Autodesk Inventor part; units mm, degrees
ref_plane "YZ Plane" through (0, 0, 0) normal (1, 0, 0) x (0, 1, 0)
ref_plane "XZ Plane" through (0, 0, 0) normal (0, 1, 0) x (-1, 0, 0)
ref_plane "XY Plane" through (0, 0, 0) normal (0, 0, 1) x (1, 0, 0)
sketch "Sketch1" plane through (0, 0, 0) normal (0, 0, 1) x (0, 1, 0)
  circle A0 centre (103.8572, -128.4288) radius 17.5
  circle A1 centre (-46.1428, 47.5712) radius 30
  circle A2 centre (-36.5428, 154.0712) radius 17.5
  arc A3 (-12.2627, 179.2798) -> (-68.6436, 140.1233) centre (-36.5428, 154.0712) ccw
  arc A4 (-79.1765, 78.1289) -> (-52.7383, 3.0571) centre (-46.1428, 47.5712) ccw
  arc A5 (68.91, -130.351) -> (138.7018, -131.7234) centre (103.8572, -128.4288) ccw
  arc A6 (239.3875, 30.5679) -> (230.7678, 67.4797) centre (228.8572, 47.5712) ccw
  arc A7 (-79.1765, 78.1289) -> (-68.6436, 140.1233) centre (-121.4095, 117.1964) ccw
  arc A8 (68.91, -130.351) -> (-52.7383, 3.0571) centre (-73.6667, -138.1931) ccw
  arc A9 (239.3875, 30.5679) -> (138.7018, -131.7234) centre (352.4092, -151.9293) ccw
  arc A10 (-12.2627, 179.2798) -> (230.7678, 67.4797) centre (269.5808, 471.9005) ccw
  dimension "d0" = 106.5
  dimension "d1" = 176
  dimension "d2" = 150
  dimension "d3" = 9.6
  dimension "d4" = 275
  dimension "d5" = 60
  dimension "d6" = 35
  dimension "d7" = 35
  dimension "d8" = 35
  dimension "d9" = 35
  dimension "d10" = 45
  dimension "d11" = 20
extrude "Extrusion1" add sketch "Sketch1" along normal blind 10
properties part number "3136 1133 85" material "Steel, Mild"
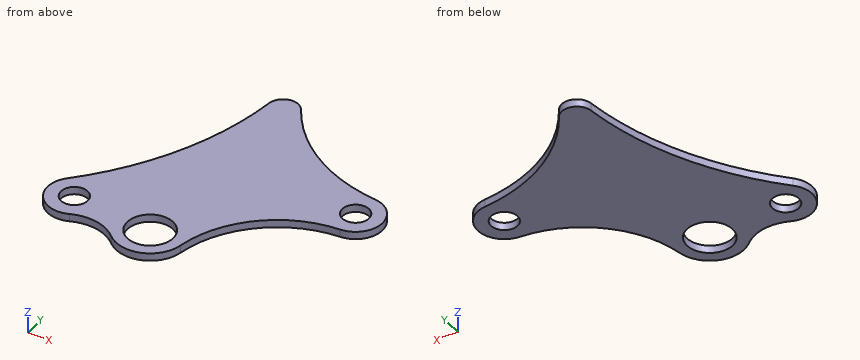
Model file for the job. Use its own axes, mm. Give positions to 0.01 mm unless a question says otherwise; leave off trailing zeros. Order: outer loops, then holes, each group sorted by start corner. A loop starts at its lowest first (then second) coordinate and runs counter-clockwise, first axis right, second up. Notation, with made-up numbers: M -14.75,2 L 42.25,2 A13 ccw 42.25,13 Z; hole C 11,1.5 d1. An arc over 180 degrees is marked long. Put each result on its own line as item: value. Start each with the question number.
(1) Band-saw the part on A-A on x = -161. Give the cut face in (y, z), then the cut area to 3 significant figures.
(2) Band-saw the part on C-C on y = 211. Give the cut face in (x, z).
(3) Band-saw the part on B-B on z = 1.5. Give the cut face in (x, y), then the cut area to 3 significant figures.
(4) Band-saw the part on D-D on x = 101. Give the cut face in (y, z).
(5) Drill centre lines: L1, parallel to X at y = -29.5, z = 9.25; L2, parallel to X at y = -52.5, z = 4; L3, parallel to Y at x = 120, z = 8.75. Where is each one in solid material? Low to high. Write a range as [from, to].
(6) Pin check, flat tips, straight feed: pin 1 Ø5 at (y, z) = (205, 5) entering from -X; pin 2 Ø1 at (x, z) = (63.5, 3) entering from +Y; pin 3 Ø1.5 at (y, z) = (128.5, 2) entering from +X. Stop position of each tip, or through.
Results below:
1. outline: M -70.85,0 L -52.61,0 L -52.61,10 L -70.85,10 Z; M -20.47,0 L 8.04,0 L 8.04,10 L -20.47,10 Z
1. area: 468 mm2
2. outline: M -69.87,0 L -9.57,0 L -9.57,10 L -69.87,10 Z
3. outline: M -179.28,-12.26 A35 ccw -140.12,-68.64 A57.53 cw -78.13,-79.18 A45 ccw -3.06,-52.74 A142.79 cw 130.35,68.91 A35 ccw 131.72,138.7 A214.66 cw -30.57,239.39 A20 ccw -67.48,230.77 A406.28 cw Z; hole C -154.07,-36.54 d35; hole C -47.57,-46.14 d60; hole C 128.43,103.86 d35
3. area: 50,300 mm2
4. outline: M 64.2,0 L 143.88,0 L 143.88,10 L 64.2,10 Z
5. L1: x = [-188.36, -170.09], [-138.05, -72.53], [-22.61, 2.4]
5. L2: x = [-185.22, -161.26], [-146.89, -76.89], [-18.25, -3.02]
5. L3: y = [67.96, 88.52], [119.19, 140.14]
6. pin 1: stops at x = -71.2
6. pin 2: stops at y = 157.04
6. pin 3: stops at x = 154
